from build123d import *

# Parameters (mm, degrees)
F0_W     = 40
F0_H     = 40
F1_DEPTH = 2
F2_R     = 2
F2_R_2   = 3
F2_R_3   = 4
F2_W     = 10
F2_H     = 10
F3_DEPTH = 2
F4_R     = 10
F5_SIZE  = 5
F6_R     = 5
F7_DEPTH = 20
F8_SIZE  = 0.3


with BuildPart() as f1:
    # F0 (on Top) → F1 (new body)
    with BuildSketch(Plane.XY):
        Rectangle(F0_W, F0_H)
    extrude(amount=F1_DEPTH)

    # F2 (on face) → F3 (cut, through all)
    with BuildSketch(Plane.XY.offset(2)):
        with Locations((-12.800124, 10)):
            Circle(F2_R)
        with Locations((0, 10)):
            Circle(F2_R_2)
        with Locations((12.410274, 10)):
            Circle(F2_R_3)
        with Locations((-10, -10)):
            Rectangle(F2_W, F2_H)
        Polygon((12.308161, -4.941213), (6.534659, -4.941213), (3.647907, -9.941213), (6.534659, -14.941213), (12.308161, -14.941213), (15.194913, -9.941213), align=None)
    extrude(amount=-F3_DEPTH, mode=Mode.SUBTRACT)

    # F4
    f4_edges = [f1.edges().sort_by_distance(p)[0] for p in [
        (-20, 20, 1),
    ]]
    fillet(f4_edges, radius=F4_R)

    # F5
    f5_edges = [f1.edges().sort_by_distance(p)[0] for p in [
        (20, 20, 1),
    ]]
    chamfer(f5_edges, length=F5_SIZE)

    # F6 (on face) → F7 (join)
    with BuildSketch(Plane.XY.offset(2)):
        Circle(F6_R)
    extrude(amount=F7_DEPTH)

    # F8
    f8_edges = [f1.edges().sort_by_distance(p)[0] for p in [
        (2.5, 20, 0),
        (17.5, 17.5, 0),
        (-17.071068, 17.071068, 0),
        (20, -2.5, 0),
        (-20, -5, 0),
        (0, -20, 0),
        (-10, -5, 0),
        (-15, -10, 0),
        (-10, -15, 0),
        (-5, -10, 0),
        (9.42141, -4.941213, 0),
        (5.091283, -7.441213, 0),
        (5.091283, -12.441213, 0),
        (9.42141, -14.941213, 0),
        (13.751537, -12.441213, 0),
        (13.751537, -7.441213, 0),
        (-14.800124, 10, 0),
        (-3, 10, 0),
        (8.410274, 10, 0),
    ]]
    chamfer(f8_edges, length=F8_SIZE)


solid = f1.part
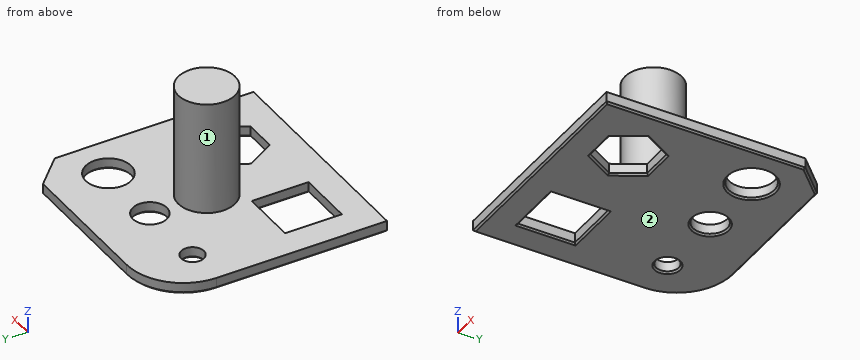
CAD build for the part. Positions are in the model's coordinates, mm. Face numbers are marked on the shaded views. A direction names the side the tool comes from. Give positions to 0.01 mm unless a question says otherwise; leave off trailing zeros. Write each loop counter-clockwise with the first axis right and the second up, starting at its lowest first coordinate (ties: lowest second). Pieces come first, ordered by that corner, then holes. Notation, with made-up numbers: (36.25, 63.5) -> (66.25, 63.5) arc R15 ccw to (66.25, 74.5) -> close; hole circle Ø7 at (22, 42). An arc over 180 degrees is marked (long way). Return JSON: item names as keys, results as strings.
Item 1: Tool access for the marked faces 1 and 2: list every direction of +Z, -Z, +X, -X, +Y, -Y with a clear straight run to the whole face (end or side of a thin tool).
Answer below:
{"face 1": "+Z", "face 2": "-Z, +X, -X, +Y, -Y"}
Item 2: Band-saw the part on A-A (x = 0). List the corners of the cut face in (y, z), then the cut area to 3 significant figures.
Answer below:
{"outline": "(-20, 0.3) -> (-19.7, 0) -> (6.7, 0) -> (7, 0.3) -> (7, 2) -> (5, 2) -> (5, 22) -> (-5, 22) -> (-5, 2) -> (-20, 2) -> close; (13, 0.3) -> (13.3, 0) -> (19.7, 0) -> (20, 0.3) -> (20, 2) -> (13, 2) -> close", "area": "268 mm2"}
Item 3: Band-saw the part on D-D (x = -9). List the corners of the cut face in (y, z), then the cut area to 3 significant figures.
Answer below:
{"outline": "(-20, 0.3) -> (-19.7, 0) -> (-15.3, 0) -> (-15, 0.3) -> (-15, 2) -> (-20, 2) -> close; (-5, 0.3) -> (-4.7, 0) -> (19.7, 0) -> (20, 0.3) -> (20, 2) -> (-5, 2) -> close", "area": "59.8 mm2"}
Item 4: Band-saw the part on B-B (y = -10.5). List the corners of the cut face in (x, z), then the cut area to 3 significant figures.
Answer below:
{"outline": "(-20, 0.3) -> (-19.7, 0) -> (-15.3, 0) -> (-15, 0.3) -> (-15, 2) -> (-20, 2) -> close; (-5, 0.3) -> (-4.7, 0) -> (3.62, 0) -> (3.97, 0.3) -> (3.97, 2) -> (-5, 2) -> close; (14.87, 0.3) -> (15.22, 0) -> (19.7, 0) -> (20, 0.3) -> (20, 2) -> (14.87, 2) -> close", "area": "37.9 mm2"}
Item 5: Drop flat-ended pins along their axis: pin 1 (7 mm diameter, centred on x = 0, y = 10, fed in from +Z); pin 2 (4 mm diameter, centred on x = -5, z = 10.5, fed in from -Y); pin 3 (1 mm diameter, centred on y = 1.5, z = 11, fed in from -X). Give the stop position or say it passes through.
Answer below:
{"pin 1": "stops at z = 2", "pin 2": "stops at y = -4", "pin 3": "stops at x = -4.9"}
Item 6: Drill centre lines: probe 1 along Y at (x, z) = (0, 1.5); probe 2 along Z at (x, y) = (-4.5, 6); probe 3 along Y at (x, z) = (-1.5, 10.25). Where is each one in solid material? Low to high.
Answer below:
{"probe 1": "y = -20 to 7, 13 to 20", "probe 2": "z = 0 to 2", "probe 3": "y = -4.77 to 4.77"}
Item 7: Band-saw the part on C-C (y = 0). List the corners of the cut face in (x, z), then the cut area to 3 significant figures.
Answer below:
{"outline": "(-20, 0.3) -> (-19.7, 0) -> (19.7, 0) -> (20, 0.3) -> (20, 2) -> (5, 2) -> (5, 22) -> (-5, 22) -> (-5, 2) -> (-20, 2) -> close", "area": "280 mm2"}
